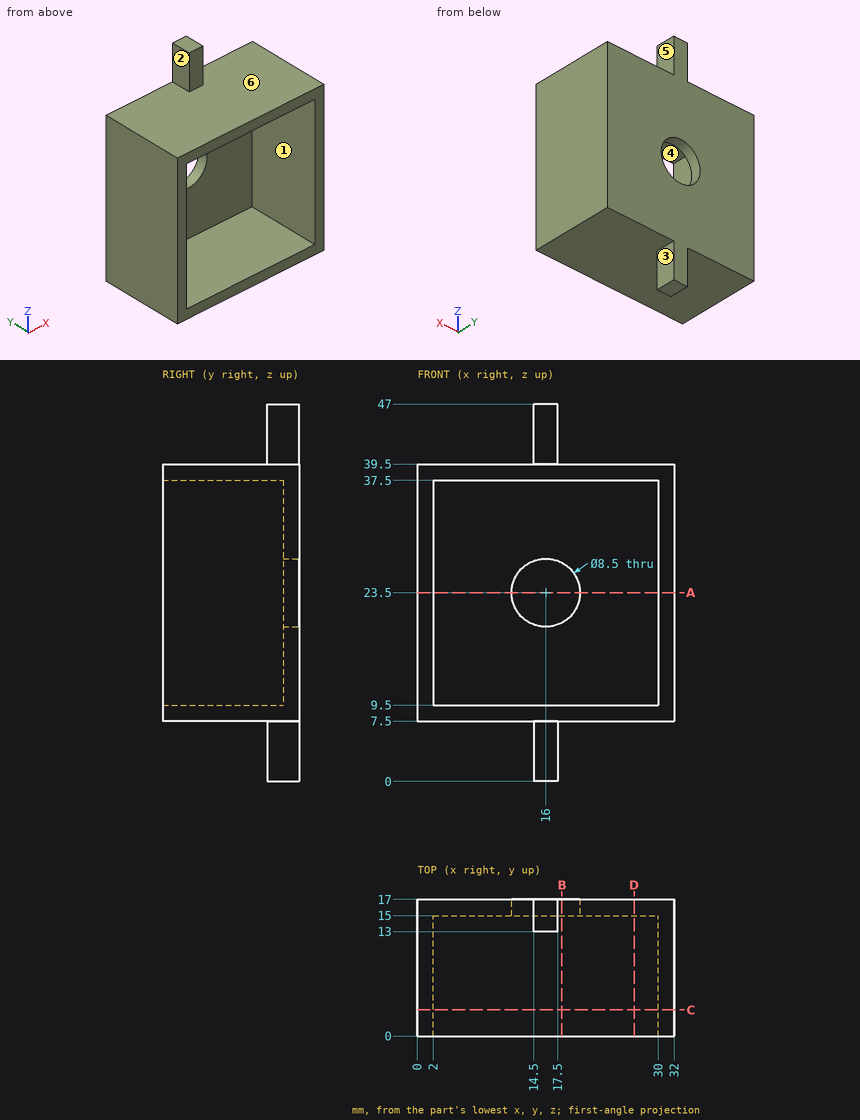
Part print with two shaded views. Sizes in mm from the minimum x, y, z corner. A direction names the side the tool comes from. Coordinates: 2 decimals unless noted, no trailing zeros. Write each loop counter-clockwise with the first axis right and the second up, starting at its lowest first coordinate (ties: lowest second). Pieces come first, ordered by that corner, then holes.
1. Band-saw the part on A-A, the plane z = 23.5. Give the cut face in (x, y), and give its area (3 significant figures).
Answer block:
outline: (0, 0) - (2, 0) - (2, 15) - (11.75, 15) - (11.75, 17) - (0, 17) - close; (20.25, 15) - (30, 15) - (30, 0) - (32, 0) - (32, 17) - (20.25, 17) - close
area: 107 mm2
2. Band-saw the part on C-C, the plane y = 3.25. Give the cut face in (x, z), and give its area (3 significant figures).
Answer block:
outline: (0, 7.5) - (32, 7.5) - (32, 39.5) - (0, 39.5) - close; hole (2, 9.5) - (30, 9.5) - (30, 37.5) - (2, 37.5) - close
area: 240 mm2
3. 3-axis set-ups, long thin cutter, end or side, ignore diameter. For the marked faces 1, 2 and 3: which of +Z, -Z, +X, -X, +Y, -Y reach the whole face in a straight line?
Answer block:
face 1: -Y
face 2: +Z, -X, +Y, -Y
face 3: -Z, +X, +Y, -Y
4. Drop flat-ended pins along their axis: pin 1 (1.5 mm diameter, centred on x = 6, y = 4.5, fed in from -Z); pin 2 (5 mm diameter, centred on x = 23.5, y = 9.5, fed in from +Z); pin 3 (8.5 mm diameter, centred on x = 13.5, z = 19.5, fed in from -Y); pin 4 (7 mm diameter, centred on x = 16, z = 23.5, fed in from -Y). Give the stop position or say it passes through.
Answer block:
pin 1: stops at z = 7.5
pin 2: stops at z = 39.5
pin 3: stops at y = 15
pin 4: passes through
5. Band-saw the part on D-D, the plane x = 27. Give the cut face in (y, z), and give its area (3 significant figures).
Answer block:
outline: (0, 7.5) - (17, 7.5) - (17, 39.5) - (0, 39.5) - (0, 37.5) - (15, 37.5) - (15, 9.5) - (0, 9.5) - close
area: 124 mm2
6. Drill centre lines: probe 1 along Z at (x, y) = (25.5, 6); probe 2 along Z at (x, y) = (16, 16.2); probe 3 along X at (y, z) = (10.75, 10). Where is each one in solid material? Low to high.
Answer block:
probe 1: z = 7.5 to 9.5, 37.5 to 39.5
probe 2: z = 0 to 19.25, 27.75 to 47
probe 3: x = 0 to 2, 30 to 32
7. Band-saw the part on B-B, the plane x = 18. Give the cut face in (y, z).
Answer block:
outline: (0, 7.5) - (17, 7.5) - (17, 19.75) - (15, 19.75) - (15, 9.5) - (0, 9.5) - close; (0, 37.5) - (15, 37.5) - (15, 27.25) - (17, 27.25) - (17, 39.5) - (0, 39.5) - close
8. Pull direction X, two halves, no side cores. Call the marked faces 4, 5 and 6: released by +X, released by -X, zero draft, split by the parting line, or undercut.
Answer block:
face 4: undercut
face 5: released by +X
face 6: zero draft
